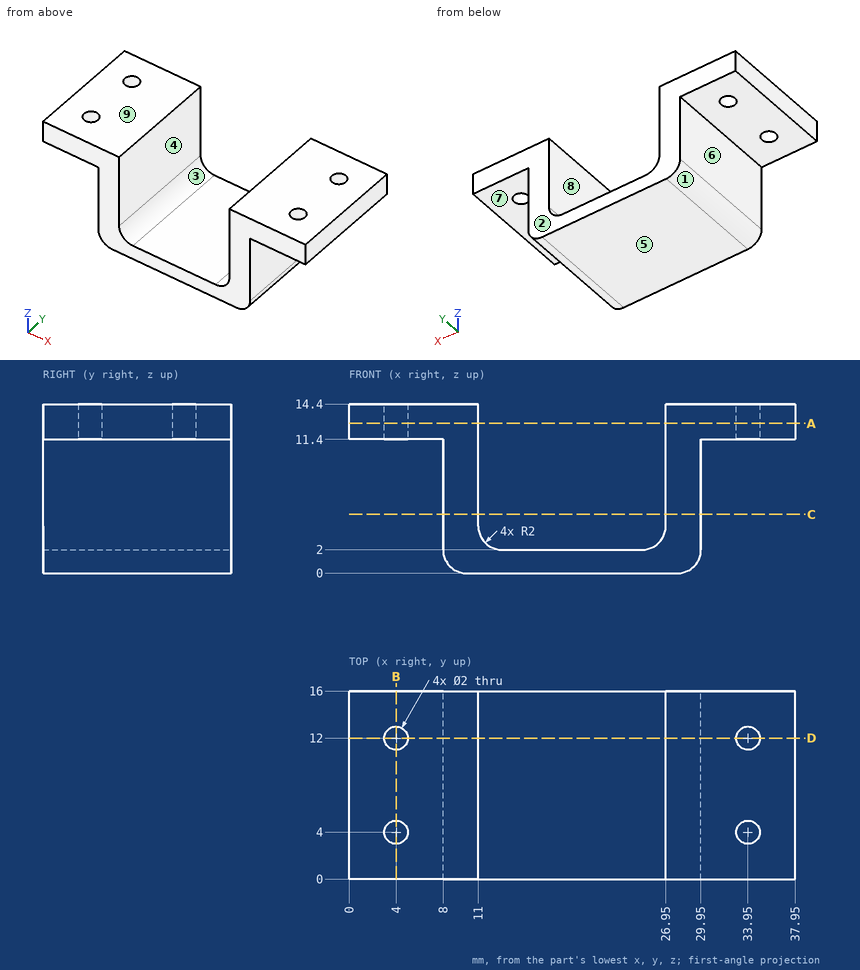
Check sheet for the drawn part. Datum: minimum x, y, z corner. Units: mm. A direction names the side the tool comes from. Round coordinates to 2 decimals unless told otherwise and drop trailing zeros. Order: outer loops, then holes, each group sorted by start corner. A loop starts at its lowest first (then second) coordinate and runs counter-clockwise, first axis right, second up.
1) Section check C-C (z = 5). Record the boundary of the cut face in (x, y).
2) Section check A-A (z = 12.75). Record the boundary of the cut face in (x, y).
3) Go/stop test with flat-tipped pins: pin 1 Ø9 at (x, y) = (33.5, 12) entering from -Z; pin 2 Ø6 at (x, y) = (20.5, 5) entering from +Z; pin 3 Ø5 at (y, z) = (12.5, 6.5) entering from +X. Record where each tip stops, or that it passes through.
4) Section check D-D (y = 12). Record the boundary of the cut face in (x, z), and give its area (3 significant figures).
5) Section check B-B (x = 4). Record the boundary of the cut face in (y, z), and give its area (3 significant figures).
6) Tool access check on the marked faces 5, 6, 7, 8 and 9. Record the directions out of +Z, -Z, +X, -X, +Y, -Y that give a thin tool (end or side, any length) a straight path to the whole face; none if there is none.
7) Scan lines: line 1 (Y direction, x = 33.95, z = 13.3); line 2 (X direction, y = 5.5, z = 7.5); line 3 (X direction, y = 2.25, z = 13.25). Record each from-to range of solid material in increasing order.
8) Mould release check, pull along X, two halves, no side actions. Record for the marked faces 1, 2, 3 and 4: +X half, -X half, draft (parallel to the pull), parting line (faces both ways), or undercut.
Result:
1. outline: (8, 0) - (11, 0) - (11, 16) - (8, 16) - close; (26.95, 0) - (29.95, 0) - (29.95, 16) - (26.95, 16) - close
2. outline: (0, 0) - (11, 0) - (11, 16) - (0, 16) - close; (26.95, 0) - (37.95, 0) - (37.95, 16) - (26.95, 16) - close; hole circle Ø2 at (4, 4); hole circle Ø2 at (4, 12); hole circle Ø2 at (33.95, 4); hole circle Ø2 at (33.95, 12)
3. pin 1: stops at z = 0.3
3. pin 2: stops at z = 2
3. pin 3: stops at x = 29.95
4. outline: (0, 11.4) - (3, 11.4) - (3, 14.4) - (0, 14.4) - close; (5, 11.4) - (8, 11.4) - (8, 2) arc R2 ccw to (10, 0) - (27.95, 0) arc R2 ccw to (29.95, 2) - (29.95, 11.4) - (32.95, 11.4) - (32.95, 14.4) - (26.95, 14.4) - (26.95, 4) arc R2 cw to (24.95, 2) - (13, 2) arc R2 cw to (11, 4) - (11, 14.4) - (5, 14.4) - close; (34.95, 11.4) - (37.95, 11.4) - (37.95, 14.4) - (34.95, 14.4) - close
4. area: 154 mm2
5. outline: (0, 11.4) - (3, 11.4) - (3, 14.4) - (0, 14.4) - close; (5, 11.4) - (11, 11.4) - (11, 14.4) - (5, 14.4) - close; (13, 11.4) - (16, 11.4) - (16, 14.4) - (13, 14.4) - close
5. area: 36.0 mm2
6. face 5: -Z, +X, -X, +Y, -Y
6. face 6: -Z, -X, +Y, -Y
6. face 7: -Z, +X, +Y, -Y
6. face 8: +Z, +Y, -Y
6. face 9: +Z, +X, -X, +Y, -Y
7. line 1: y = 0 to 3, 5 to 11, 13 to 16
7. line 2: x = 8 to 11, 26.95 to 29.95
7. line 3: x = 0 to 11, 26.95 to 37.95
8. face 1: -X half
8. face 2: draft
8. face 3: undercut
8. face 4: undercut
